from build123d import *

# Parameters (mm, degrees)
SKETCH1_W           = 112
SKETCH1_H           = 95.35
BOSS_EXTRUDE1_DEPTH = 3.175
SKETCH2_W           = 40
SKETCH2_H           = 3.175
SKETCH2_W_2         = 26
CUT_EXTRUDE1_DEPTH  = 74.613763998
SKETCH4_W           = 10
SKETCH4_H           = 3.175
BOSS_EXTRUDE2_DEPTH = 3.175
SKETCH5_W           = 10
SKETCH5_H           = 3.175
BOSS_EXTRUDE3_DEPTH = 3.175


with BuildPart() as part:
    # Sketch1 → Boss-Extrude1 (new body)
    with BuildSketch(Plane(origin=(0, 0, 0), x_dir=(1, 0, 0), z_dir=(0, 1, 0))):
        Rectangle(SKETCH1_W, SKETCH1_H)
    extrude(amount=BOSS_EXTRUDE1_DEPTH)

    # Sketch2 → Cut-Extrude1 (cut, through all)
    with BuildSketch(Plane(origin=(0, 3.175, 0), x_dir=(1, 0, 0), z_dir=(0, 1, 0))):
        with Locations((0, 46.0875)):
            Rectangle(SKETCH2_W, SKETCH2_H)
        with Locations((43, 46.0875)):
            Rectangle(SKETCH2_W_2, SKETCH2_H)
        with Locations((-43, 46.0875)):
            Rectangle(SKETCH2_W_2, SKETCH2_H)
        with Locations((0, -46.0875)):
            Rectangle(SKETCH2_W, SKETCH2_H)
        with Locations((-43, -46.0875)):
            Rectangle(SKETCH2_W_2, SKETCH2_H)
        with Locations((43, -46.0875)):
            Rectangle(SKETCH2_W_2, SKETCH2_H)
    extrude(amount=-CUT_EXTRUDE1_DEPTH, mode=Mode.SUBTRACT)

    # Sketch4 → Boss-Extrude2 (add)
    with BuildSketch(Plane.ZY.offset(56)):
        with Locations((0, 1.5875)):
            Rectangle(SKETCH4_W, SKETCH4_H)
    extrude(amount=BOSS_EXTRUDE2_DEPTH)

    # Sketch5 → Boss-Extrude3 (add)
    with BuildSketch(Plane(origin=(56, 0, 0), x_dir=(0, 0, -1), z_dir=(1, 0, 0))):
        with Locations((0, 1.5875)):
            Rectangle(SKETCH5_W, SKETCH5_H)
    extrude(amount=BOSS_EXTRUDE3_DEPTH)


solid = part.part
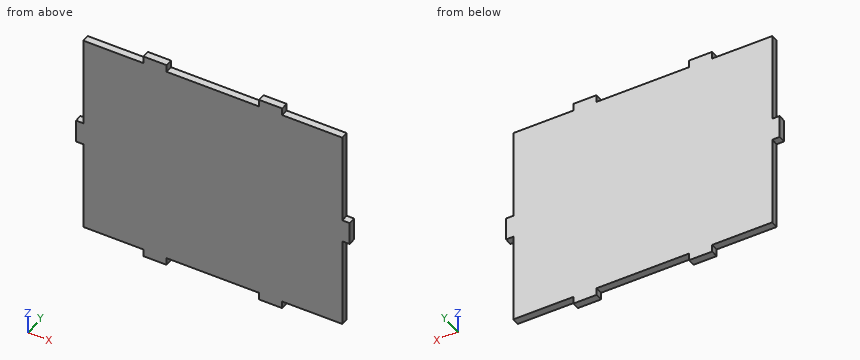
Geometry: final body of the model. Coordinates: model frame, mm. Coordinates: 2 decimals unless noted, no trailing zeros. Loops run counter-clockwise (first coordinate to the right, second up) from the corner with the lowest first, then second, coordinate; pieces in that order, holes last. Notation, with made-up numbers: M 87.25,-13.75 L 140.25,-13.75 A13 cw 140.25,0.25 Z; hole C -8.5,63 d3. An arc over 180 degrees is marked long. One line per item, written item: value. Start each with the question number.
1) Pin query (flat end, axial travel): P1, Ø1.6, axis at y = 2.5, z = -46.5, coming from the +X side; P2, Ø1.5, axis at x = 8, y = 1, coming from the -Z side; P3, Ø1.6, axis at x = 57, y = 1, coming from the +Z side. Return the tip coordinate at first contact, or that it passes through.
2) Material intervals for L1, parallel to X at y = 0.7, z = -15.5; L2, parallel to Z at x = -13, y = 1.6, sorted ascending. Write a range as from..to.
3) Cut plane B-B (x = 42). Return loops of the section in (y, z) (3 decimals), then the cut area to 3 significant figures.
4) Cut plane C-C (z = 26.5). Return loops of the section in (x, y) (3 decimals), then the cut area to 3 significant figures.
5) Cut plane A-A (y = 2). Return loops of the section in (x, z) (3 decimals), then the cut area to 3 significant figures.
Evaluation:
1. P1: x = 30
1. P2: z = -44.5
1. P3: z = 5
2. L1: -56..56
2. L2: -44.5..44.5
3. outline: M 0,-44.5 L 3.175,-44.5 L 3.175,44.5 L 0,44.5 Z
3. area: 283 mm^2
4. outline: M -56,0 L 56,0 L 56,3.175 L -56,3.175 Z
4. area: 356 mm^2
5. outline: M -59.175,-5 L -56,-5 L -56,-44.5 L -30,-44.5 L -30,-47.675 L -20,-47.675 L -20,-44.5 L 20,-44.5 L 20,-47.675 L 30,-47.675 L 30,-44.5 L 56,-44.5 L 56,-5 L 59.175,-5 L 59.175,5 L 56,5 L 56,44.5 L 30,44.5 L 30,47.675 L 20,47.675 L 20,44.5 L -20,44.5 L -20,47.675 L -30,47.675 L -30,44.5 L -56,44.5 L -56,5 L -59.175,5 Z
5. area: 10,200 mm^2
